Source: CAD feature listing. Evaluate the final solid. Frame: model axes, mm. A direction names the side the tool comes from. Round coordinates to 2 decimals unless told otherwise and drop trailing zeros. Loops run counter-clockwise (first coordinate to the right, second up) from the corner with the lowest first, then second, coordinate; pieces in that order, holes last.
Item 1: Pull-direction query (X, two-part tool) for faces 4 (the cylindrical face through (13.858, -10.626, -21.424)), 5 (the flat face through (6, -3, 20.638)), 6 (the flat face through (-5.474, -3.219, -1.094)); classes: released by +X, released by -X, zero draft, split by the parting line, or undercut.
Item 2: First-contact query: P1, Ø10, axis at x = 6.5, z = -5, coming from the +Y side; P2, Ø4, axis at x = 10, y = -13, coming from the +Z side; P3, Ø8, axis at y = -8.5, z = 1, coming from the +X side. Flat tips, straight axial feed; report the tip coordinate or a pass-through.
Item 3: Access query for faces 1 (the cylindrical face through (-3.3, -14.88, -0.52)), 2 (the flat face through (-7.4, 0.2, -22.225)), 3 (the flat face through (5.474, 3.219, -1.094)). Directions: +Z, -Z, +X, -X, +Y, -Y. A direction counts if a zero-diameter tool reaches every point of the face in a straight line with its end or side. Return the directions, or none.
Item 4: Section query B-B on z = -6.5. Return loops of the section in (x, y).
Item 5: Ray query, L1, parallel to Z at x = -10.5, y = -12 (1 decimal); L2, parallel to X at y = -6, z = 6.5; L3, parallel to Y at x = -1, z = -4. Return the intervals inside material, ascending.
```python
from build123d import *

# Parameters (mm, degrees)
SKETCH1_R           = 15.24
BOSS_EXTRUDE1_DEPTH = 20.6375
CHAMFER1_SIZE       = 1.5875
SKETCH2_R           = 17.4625
BOSS_EXTRUDE2_DEPTH = 1.5875
CUT_EXTRUDE1_DEPTH  = 50.467885732
CHAMFER2_SIZE       = 0.254


with BuildPart() as part:
    # Sketch1 → Boss-Extrude1 (new, symmetric)
    with BuildSketch(Plane.XY):
        Circle(SKETCH1_R)
    extrude(amount=BOSS_EXTRUDE1_DEPTH, both=True)

    # Chamfer1
    chamfer1_edges = [part.edges().sort_by_distance(p)[0] for p in [
        (-15.24, 0, 20.6375),
    ]]
    chamfer(chamfer1_edges, length=CHAMFER1_SIZE)

    # Sketch2 → Boss-Extrude2 (add)
    with BuildSketch(Plane(origin=(0, 0, -20.6375), x_dir=(-1, 0, 0), z_dir=(0, 0, -1))):
        Circle(SKETCH2_R)
    extrude(amount=BOSS_EXTRUDE2_DEPTH)

    # Sketch3 → Cut-Extrude1 (cut, through all)
    with BuildSketch(Plane(origin=(0, 0, -22.225), x_dir=(-1, 0, 0), z_dir=(0, 0, -1))):
        Polygon((7.332348419, 0), (3.666174209, 6.35), (-3.666174209, 6.35), (-7.332348419, 0), (-3.666174209, -6.35), (3.666174209, -6.35), align=None)
    extrude(amount=-CUT_EXTRUDE1_DEPTH, mode=Mode.SUBTRACT)

    # Chamfer2
    chamfer2_edges = [part.edges().sort_by_distance(p)[0] for p in [
        (17.4625, 0, -20.6375),
        (17.4625, 0, -22.225),
    ]]
    chamfer(chamfer2_edges, length=CHAMFER2_SIZE)


solid = part.part
```
Data:
1. face 4: split by the parting line
1. face 5: zero draft
1. face 6: undercut
2. P1: stops at y = 15.17
2. P2: stops at z = 19.89
2. P3: stops at x = 14.56
3. face 1: +Z
3. face 2: -Z, +X, -X, +Y, -Y
3. face 3: +Z, -Z
4. outline: circle Ø30.48 at (0, 0); hole (-7.33, 0) - (-3.67, -6.35) - (3.67, -6.35) - (7.33, 0) - (3.67, 6.35) - (-3.67, 6.35) - close
5. L1: z = -22.2 to -20.6
5. L2: x = -14.01 to -3.87, 3.87 to 14.01
5. L3: y = -15.21 to -6.35, 6.35 to 15.21
